from build123d import *

# Parameters (mm, degrees)
SKETCH006_W      = 9.472441
SKETCH006_H      = 23
EXTRUDE005_DEPTH = 40
SKETCH005_R      = 5.5
EXTRUDE004_DEPTH = 10.25
SKETCH004_R      = 6.25
EXTRUDE003_DEPTH = 11.75
SKETCH003_R      = 7
EXTRUDE002_DEPTH = 13.1
SKETCH002_R      = 8.925
EXTRUDE001_DEPTH = 14.55
FACE_W           = 23
FACE_H           = 79.822441
EXTRUDE_DEPTH    = 30


with BuildPart() as extrude005:
    # Sketch006 (on Face5 of Cut003) → Extrude005 (new body)
    with BuildSketch(Plane.XY.offset(30)):
        with Locations((75.08622, 11.5)):
            Rectangle(SKETCH006_W, SKETCH006_H)
    extrude(amount=-EXTRUDE005_DEPTH)


with BuildPart() as extrude004:
    # Sketch005 (on Face5 of Cut002) → Extrude004 (new body)
    with BuildSketch(Plane.XY.offset(30)):
        with Locations((61.85, 11.5)):
            Circle(SKETCH005_R)
    extrude(amount=-EXTRUDE004_DEPTH)


with BuildPart() as extrude003:
    # Sketch004 (on Face5 of Cut001) → Extrude003 (new body)
    with BuildSketch(Plane.XY.offset(30)):
        with Locations((47.1, 11.5)):
            Circle(SKETCH004_R)
    extrude(amount=-EXTRUDE003_DEPTH)


with BuildPart() as extrude002:
    # Sketch003 (on Face5 of Cut) → Extrude002 (new body)
    with BuildSketch(Plane.XY.offset(30)):
        with Locations((30.85, 11.5)):
            Circle(SKETCH003_R)
    extrude(amount=-EXTRUDE002_DEPTH)


with BuildPart() as extrude001:
    # Sketch002 (on Face6 of Extrude) → Extrude001 (new body)
    with BuildSketch(Plane.XY.offset(30)):
        with Locations((11.925, 11.5)):
            Circle(SKETCH002_R)
    extrude(amount=-EXTRUDE001_DEPTH)


with BuildPart() as cut004:
    # Face → Extrude (new body)
    with BuildSketch(Plane(origin=(39.91122, 11.5, 0), x_dir=(0, 1, 0), z_dir=(0, 0, 1))):
        with Locations((0, 0)):
            Rectangle(FACE_W, FACE_H)
    extrude(amount=EXTRUDE_DEPTH)

    # Cut: cut Extrude001
    add(extrude001.part, mode=Mode.SUBTRACT)

    # Cut001: cut Extrude002
    add(extrude002.part, mode=Mode.SUBTRACT)

    # Cut002: cut Extrude003
    add(extrude003.part, mode=Mode.SUBTRACT)

    # Cut003: cut Extrude004
    add(extrude004.part, mode=Mode.SUBTRACT)

    # Cut004: cut Extrude005
    add(extrude005.part, mode=Mode.SUBTRACT)


solid = cut004.part
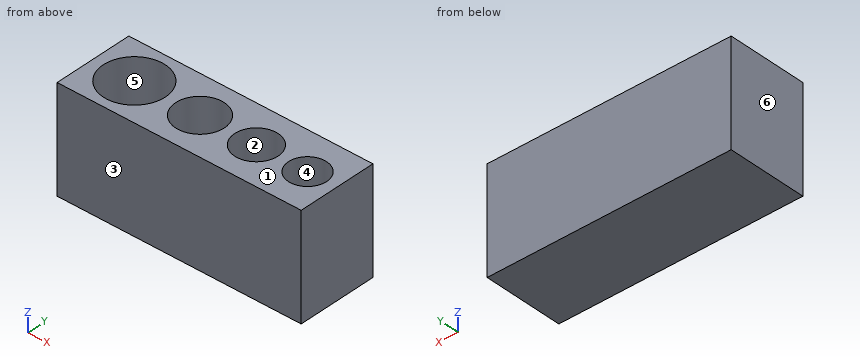
Geometry check sheet. Reference: the model listing, model coordinates, mm. Face numbers are marked on the shaded views. A direction names the side the tool comes from. Give positions to 0.01 mm unless a question says otherwise; leave off trailing zeros. Order: outer loops, then holes, each group sorted by start corner. A loop starts at its lowest first (then second) coordinate and runs counter-clockwise, first axis right, second up. Notation, with made-up numbers: (22, 35) - (34, 35) arc R24 ccw to (34, 62) - close; hole circle Ø9 at (-5, 13). An arc over 180 degrees is marked (long way). Answer as a JSON object with one key per item and string values.
(1) Tool access check on the marked faces 1 and 2. Record the directions out of +Z, -Z, +X, -X, +Y, -Y that give a thin tool (end or side, any length) a straight path to the whole face; none if there is none.
Report:
{"face 1": "+Z, +X, -X, +Y, -Y", "face 2": "+Z"}
(2) Cross-section at B-B (x = 47.1). Record the cut outline in (y, z).
Report:
{"outline": "(0, 0) - (23, 0) - (23, 30) - (17.75, 30) - (17.75, 18.25) - (5.25, 18.25) - (5.25, 30) - (0, 30) - close"}
(3) Material ranges on line 1 (X direction, y = 11, z = 19.5); line 2 (Y direction, x = 61.85, z = 28.25); line 3 (Y direction, x = 30.85, z = 20.25), recorded low to high.
Report:
{"line 1": "0 to 3.01, 20.84 to 23.87, 37.83 to 40.87, 53.33 to 70.35", "line 2": "0 to 6, 17 to 23", "line 3": "0 to 4.5, 18.5 to 23"}
(4) Draft check along X on the marked faces 3, 4, 5 and 6. Enter one of: released by +X, released by -X, zero draft, split by the parting line, or undercut.
Report:
{"face 3": "zero draft", "face 4": "undercut", "face 5": "undercut", "face 6": "released by -X"}
(5) Cross-section at D-D (z = 16.25). Record the cut outline in (x, y) (3 decimals), then the cut area to 3 significant figures.
Report:
{"outline": "(0, 0) - (70.35, 0) - (70.35, 23) - (0, 23) - close; hole circle Ø17.85 at (11.925, 11.5)", "area": "1,370 mm^2"}
(6) Cross-section at A-A (z = 27). Record the cut outline in (x, y) (3 decimals).
Report:
{"outline": "(0, 0) - (70.35, 0) - (70.35, 23) - (0, 23) - close; hole circle Ø17.85 at (11.925, 11.5); hole circle Ø14 at (30.85, 11.5); hole circle Ø12.5 at (47.1, 11.5); hole circle Ø11 at (61.85, 11.5)"}
(7) Cross-section at C-C (y = 11.5). Record the cut outline in (x, z).
Report:
{"outline": "(0, 0) - (70.35, 0) - (70.35, 30) - (67.35, 30) - (67.35, 19.75) - (56.35, 19.75) - (56.35, 30) - (53.35, 30) - (53.35, 18.25) - (40.85, 18.25) - (40.85, 30) - (37.85, 30) - (37.85, 16.9) - (23.85, 16.9) - (23.85, 30) - (20.85, 30) - (20.85, 15.45) - (3, 15.45) - (3, 30) - (0, 30) - close"}
(8) Depth check by flat-ended pin: pin 1 Ø3 at (x, y) = (61.5, 9.5) entering from +Z; pin 2 Ø6 at (x, y) = (46, 9) entering from +Z. Enter the tip coordinate at first touch or a pass-through.
Report:
{"pin 1": "z = 19.75", "pin 2": "z = 18.25"}
